Work out the finished part from the listing and answer in its coordinate system (mm). A direction names the side the tool comes from. Coordinates: 2 decimals unless noted, no trailing zeros. Write each loop counter-clockwise with the first axis right and the second up, starting at its lowest first coordinate (ties: lowest second). Pieces come first, ordered by that corner, then holes. Notation, with made-up numbers: (-0.75, 41) - (57.25, 41) arc R20 ccw to (57.25, 45) - close; hole circle Ø4 at (20, 15.25). An arc over 180 degrees is marked (long way). One line per item, written item: value.
```python
from build123d import *

# Parameters (mm, degrees)
SKETCH1_R           = 7.5
SKETCH1_R_2         = 4
BOSS_EXTRUDE1_DEPTH = 5
SKETCH3_R           = 10
SKETCH3_R_2         = 1.5
BOSS_EXTRUDE3_DEPTH = 8
BOSS_EXTRUDE4_START = 15
SKETCH4_R           = 7.5
SKETCH4_R_2         = 4
BOSS_EXTRUDE4_DEPTH = 15
SKETCH2_R           = 2
CUT_EXTRUDE1_DEPTH  = 7
SKETCH6_R           = 4
CUT_EXTRUDE2_DEPTH  = 32.368774283
BOSS_EXTRUDE5_START = 2
SKETCH7_R           = 10
SKETCH7_R_2         = 4
BOSS_EXTRUDE5_DEPTH = 2


with BuildPart() as part:
    # Sketch1 → Boss-Extrude1 (new body)
    # profile 1 of 2: a face of its own
    with BuildSketch(Plane.XY):
        Circle(SKETCH1_R)
        Circle(SKETCH1_R_2, mode=Mode.SUBTRACT)
    # profile 2 of 2: a face of its own
    with BuildSketch(Plane.XY):
        Circle(SKETCH1_R_2)
    extrude(amount=-BOSS_EXTRUDE1_DEPTH)

    # Sketch3 → Boss-Extrude3 (add)
    with BuildSketch(Plane(origin=(0, 0, -5), x_dir=(-1, 0, 0), z_dir=(0, 0, -1))):
        Circle(SKETCH3_R)
        with Locations(Location((0, 7, 0), (0, 0, 166.225853002))):
            Circle(SKETCH3_R_2, mode=Mode.SUBTRACT)
        with Locations(Location((7, 0, 0), (0, 0, 283.774146998))):
            Circle(SKETCH3_R_2, mode=Mode.SUBTRACT)
        with Locations(Location((0, -7, 0), (0, 0, 193.774146998))):
            Circle(SKETCH3_R_2, mode=Mode.SUBTRACT)
        with Locations(Location((-7, 0, 0), (0, 0, 256.225853002))):
            Circle(SKETCH3_R_2, mode=Mode.SUBTRACT)
    extrude(amount=BOSS_EXTRUDE3_DEPTH)

    # Sketch4 → Boss-Extrude4 (add)
    with BuildSketch(Plane.XY.offset(BOSS_EXTRUDE4_START)):
        Circle(SKETCH4_R)
        Circle(SKETCH4_R_2, mode=Mode.SUBTRACT)
    extrude(amount=-BOSS_EXTRUDE4_DEPTH)

    # Sketch2 → Cut-Extrude1 (cut)
    with BuildSketch(Plane(origin=(0, 7.5, 0), x_dir=(1, 0, 0), z_dir=(0, 1, 0))):
        with Locations(Location((0, -10, 0), (0, 0, 270))):
            Circle(SKETCH2_R)
    extrude(amount=-CUT_EXTRUDE1_DEPTH, mode=Mode.SUBTRACT)

    # Sketch6 → Cut-Extrude2 (cut, through all)
    with BuildSketch(Plane.XY.offset(15)):
        Circle(SKETCH6_R)
    extrude(amount=-CUT_EXTRUDE2_DEPTH, mode=Mode.SUBTRACT)

    # Sketch7 → Boss-Extrude5 (add)
    with BuildSketch(Plane.XY.offset(-5).offset(BOSS_EXTRUDE5_START)):
        Circle(SKETCH7_R)
        Circle(SKETCH7_R_2, mode=Mode.SUBTRACT)
    extrude(amount=-BOSS_EXTRUDE5_DEPTH)


solid = part.part
```
Item 1: Consider probe 1 along Y at (x, z) = (0, -9.5); probe 2 along X at (y, z) = (-1.25, -8.75); probe 3 along Y at (x, z) = (0, 2.5). Determine where each line is inside the solid, lowest interval first.
Evaluation:
probe 1: y = -10 to -8.5, -5.5 to -4, 4 to 5.5, 8.5 to 10
probe 2: x = -9.92 to -7.83, -6.17 to -3.8, 3.8 to 6.17, 7.83 to 9.92
probe 3: y = -7.5 to -4, 4 to 7.5
Item 2: Given pin 1 (5 mm diameter, centred on x = 0, z = 10, fed in from -Y); pin 2 (2.5 mm diameter, centred on x = 0, y = -7, fed in from -Z); pin 3 (4 mm diameter, centred on x = -5.5, z = 3.5, fed in from +Y); pin 4 (7 mm diameter, centred on x = 0, y = 0, fed in from +Z), each flat-ended and moving along its own axis, determine where each tip first touches the part or whether it passes through.
Evaluation:
pin 1: stops at y = -7.5
pin 2: stops at z = -5
pin 3: stops at y = 6.63
pin 4: passes through
Item 3: Section A-A, the plane y = 0 is taken. Determine the outline of the cut face in (x, z).
Evaluation:
outline: (-10, -13) - (-8.5, -13) - (-8.5, -5) - (-5.5, -5) - (-5.5, -13) - (-4, -13) - (-4, 15) - (-7.5, 15) - (-7.5, -3) - (-10, -3) - close; (4, -13) - (5.5, -13) - (5.5, -5) - (8.5, -5) - (8.5, -13) - (10, -13) - (10, -3) - (7.5, -3) - (7.5, 15) - (4, 15) - close
Item 4: Section D-D, the plane x = 6.5 is taken. Determine the outline of the cut face in (y, z), then the cut area to 3 significant figures.
Evaluation:
outline: (-7.6, -13) - (-1.41, -13) - (-1.41, -5) - (1.41, -5) - (1.41, -13) - (7.6, -13) - (7.6, -3) - (3.74, -3) - (3.74, 15) - (-3.74, 15) - (-3.74, -3) - (-7.6, -3) - close
area: 264 mm2
Item 5: Which of the six approach directions +Z, -Z, +X, -X, +Y, -Y give full straight-line access (tool end or side, diameter ignored) to faces 1 (the face through (0.355, 8.457, -8.944)), 2 (the face through (4, 7, -3)), 3 (the face through (1.686, 5.511, 11.075)), 4 (the face through (0.1, -4.3, -13))?
Evaluation:
face 1: -Z
face 2: +Z
face 3: +Y
face 4: -Z, +X, -X, +Y, -Y
Item 6: Section B-B, the plane x = 0 is taken. Determine the outline of the cut face in (y, z).
Evaluation:
outline: (-10, -13) - (-8.5, -13) - (-8.5, -5) - (-5.5, -5) - (-5.5, -13) - (-4, -13) - (-4, 15) - (-7.5, 15) - (-7.5, -3) - (-10, -3) - close; (4, -13) - (5.5, -13) - (5.5, -5) - (8.5, -5) - (8.5, -13) - (10, -13) - (10, -3) - (7.5, -3) - (7.5, 8) - (4, 8) - close; (4, 12) - (7.5, 12) - (7.5, 15) - (4, 15) - close
Item 7: Section C-C, the plane z = -8 is taken. Determine the outline of the cut face in (x, y), then the cut area to 3 significant figures.
Evaluation:
outline: circle Ø20 at (0, 0); hole circle Ø3 at (-7, 0); hole circle Ø8 at (0, 0); hole circle Ø3 at (0, -7); hole circle Ø3 at (0, 7); hole circle Ø3 at (7, 0)
area: 236 mm2
Item 8: Determine the mould class of faces 5 (the face through (-1.63, -7.32, 6.13)), 6 (the face through (-5.5, 0, -8.9)), 7 (the face through (3, -3, 15)) for opening direction Y: +Y half, -Y half, draft (parallel to the pull), parting line (faces both ways), or undercut.
Evaluation:
face 5: parting line
face 6: undercut
face 7: draft
